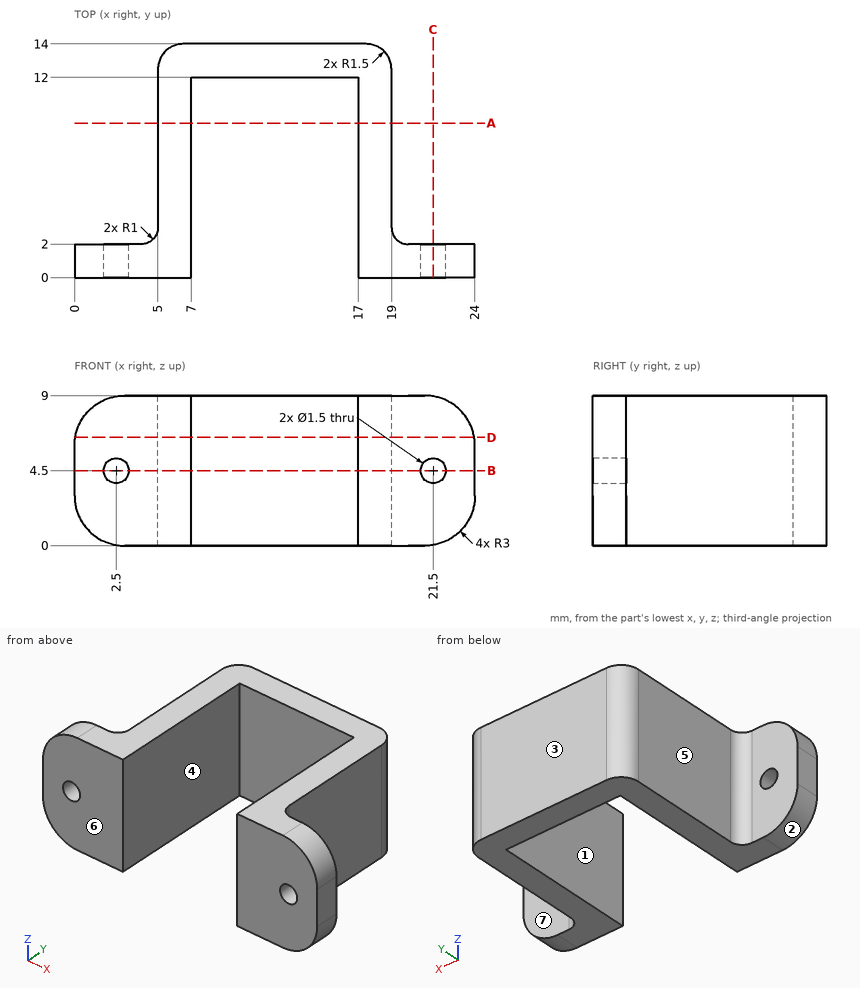
Here's the drawing with two shaded views (mm, measured from the low corner). I have some questions. A direction names the side the tool comes from. Coordinates: 2 decimals unless noted, no trailing zeros. Order: outer loops, then holes, each group sorted by start corner. A loop starts at its lowest first (then second) coordinate and runs counter-clockwise, first axis right, second up. Notation, with made-up numbers: (22.25, 46) - (52.25, 46) arc R15 ccw to (52.25, 70) - close; hole circle Ø4 at (-1.5, -14.75). An arc over 180 degrees is marked (long way). Answer in a Markdown table with one row per item. Add a question column.
(1) If we section it at D-D, the plane z = 6.5: Please give me the cut outline in (x, y), then the cut area to 3 significant figures.
(2) If we section it at A-A, the plane y = 9.25: Please give me the cut outline in (x, z), then the cut area to 3 significant figures.
(3) I need wall thicknesses on L1, parallel to X at y = 0.7, z = 4.5; L2, parallel to X at y = 5.25, z = 3; L3, parallel to X at y = 12.5, z = 7.25. Which ranges of each line are inside material? Lowest first, please.
(4) If we section it at B-B, the plane z = 4.5: Please give me the cut outline in (x, y).
(5) Will these pins go through, and if not, where does the flat tip stop? pin 1 (2 mm diameter, centred on x = 22.5, z = 2.5, fed in from +Y); pin 2 (3 mm diameter, centred on y = 8, z = 6, fed in from +X).
(6) On a 3-axis mill with a long thin cutter (end or side, diameter ignored), from which of +Z, -Z, +X, -X, +Y, -Y can I reach the whole of each face in a straight line? I mean the marked faces 4, 5, 6 and 7. Say none if no direction works.
(7) If we mould it in two halves opening along X, with no side actions, what happens to the marked faces 1, 2 and 3? For each: released by +X, released by -X, zero draft, split by the parting line, or undercut.
(8) If we section it at C-C, the plane x = 21.5: Please give me the cut outline in (y, z), then the cut area to 3 significant figures.
Results are:
| question | item | result |
|---|---|---|
| 1 | outline | (0.04, 0) - (7, 0) - (7, 12) - (17, 12) - (17, 0) - (23.96, 0) - (23.96, 2) - (20, 2) arc R1 cw to (19, 3) - (19, 12.5) arc R1.5 ccw to (17.5, 14) - (6.5, 14) arc R1.5 ccw to (5, 12.5) - (5, 3) arc R1 cw to (4, 2) - (0.04, 2) - close |
| 1 | area | 95.3 mm2 |
| 2 | outline | (5, 0) - (7, 0) - (7, 9) - (5, 9) - close; (17, 0) - (19, 0) - (19, 9) - (17, 9) - close |
| 2 | area | 36.0 mm2 |
| 3 | L1 | x = 0 to 1.75, 3.25 to 7, 17 to 20.75, 22.25 to 24 |
| 3 | L2 | x = 5 to 7, 17 to 19 |
| 3 | L3 | x = 5 to 19 |
| 4 | outline | (0, 0) - (1.75, 0) - (1.75, 2) - (0, 2) - close; (3.25, 0) - (7, 0) - (7, 12) - (17, 12) - (17, 0) - (20.75, 0) - (20.75, 2) - (20, 2) arc R1 cw to (19, 3) - (19, 12.5) arc R1.5 ccw to (17.5, 14) - (6.5, 14) arc R1.5 ccw to (5, 12.5) - (5, 3) arc R1 cw to (4, 2) - (3.25, 2) - close; (22.25, 0) - (24, 0) - (24, 2) - (22.25, 2) - close |
| 5 | pin 1 | stops at y = 2 |
| 5 | pin 2 | stops at x = 19 |
| 6 | face 4 | +Z, -Z, -Y |
| 6 | face 5 | +Z, -Z, -X, +Y |
| 6 | face 6 | +Z, -Z, +X, -X, -Y |
| 6 | face 7 | +Z, -Z, +X, +Y |
| 7 | face 1 | undercut |
| 7 | face 2 | released by -X |
| 7 | face 3 | zero draft |
| 8 | outline | (0, 0.04) - (2, 0.04) - (2, 3.75) - (0, 3.75) - close; (0, 5.25) - (2, 5.25) - (2, 8.96) - (0, 8.96) - close |
| 8 | area | 14.8 mm2 |
